```python
from build123d import *

# Parameters (mm, degrees)
F0_W      = 279.4
F0_H      = 44.45
F1_DEPTH  = 31.75
F2_W      = 165.1
F2_H      = 38.1
F3_DEPTH  = 28.575
F5_DEPTH  = 31.751
F6_W      = 6.35
F6_H      = 44.45
F7_DEPTH  = 31.75
F8_R      = 9.525
F9_R      = 5.588
F10_R     = 2.54
F11_DEPTH = 279.4
F12_W     = 25.4
F12_H     = 28.575
F12_H_2   = 12.7
F13_DEPTH = 31.751
F14_R     = 2.54
F15_DEPTH = 7.62
F16_R     = 7.9375
F17_R     = 5.08
F18_R     = 4.7625
F19_DEPTH = 17.272
F20_R     = 4.7625
F21_DEPTH = 17.272
F22_R     = 1.984375
F23_DEPTH = 41.91
F24_R     = 1.5875
F25_DEPTH = 3.175


with BuildPart() as f1:
    # F0 (on Top) → F1 (new body)
    with BuildSketch(Plane.XY):
        with Locations((139.7, 22.225)):
            Rectangle(F0_W, F0_H)
    extrude(amount=F1_DEPTH)

    # F2 (on face) → F3 (cut)
    with BuildSketch(Plane.XY.offset(31.75)):
        with Locations((139.7, 22.225)):
            Rectangle(F2_W, F2_H)
    extrude(amount=-F3_DEPTH, mode=Mode.SUBTRACT)

    # F4 (on face) → F5 (cut, through all)
    with BuildSketch(Plane(origin=(0, 0, 0), x_dir=(1, 0, 0), z_dir=(0, 0, -1))):
        with BuildLine():
            Line((127, -26.035), (209.867099, -26.025243))
            ThreePointArc((209.867099, -26.025243), (213.405749, -22.066069), (209.55, -18.415))
            Line((209.55, -18.415), (127, -18.415))
            ThreePointArc((127, -18.415), (123.19, -22.225), (127, -26.035))
        make_face()
    extrude(amount=-F5_DEPTH, mode=Mode.SUBTRACT)

    # F6 (on face) → F7 (join)
    with BuildSketch(Plane.XY.offset(31.75)):
        with Locations((3.175, 22.225)):
            Rectangle(F6_W, F6_H)
        with Locations((276.225, 22.225)):
            Rectangle(F6_W, F6_H)
    extrude(amount=F7_DEPTH)

    # F8
    f8_edges = [f1.edges().sort_by_distance(p)[0] for p in [
        (57.15, 3.175, 17.4625),
        (57.15, 41.275, 17.4625),
        (222.25, 3.175, 17.4625),
        (222.25, 41.275, 17.4625),
    ]]
    fillet(f8_edges, radius=F8_R)

    # F9
    f9_edges = [f1.edges().sort_by_distance(p)[0] for p in [
        (0, 44.45, 31.75),
        (0, 0, 31.75),
        (279.4, 44.45, 31.75),
        (279.4, 0, 31.75),
    ]]
    fillet(f9_edges, radius=F9_R)

    # F10 (on Right) → F11 (cut)
    with BuildSketch(Plane.YZ):
        with Locations((22.225, 54.61)):
            Circle(F10_R)
    extrude(amount=F11_DEPTH, mode=Mode.SUBTRACT)

    # F12 (on face) → F13 (cut, through all)
    with BuildSketch(Plane.XY.offset(31.75)):
        with Locations((28.575, 22.225)):
            Rectangle(F12_W, F12_H)
        with Locations((247.65, 22.225)):
            Rectangle(F12_W, F12_H_2)
    extrude(amount=-F13_DEPTH, mode=Mode.SUBTRACT)

    # F14 (on Right) → F15 (cut)
    with BuildSketch(Plane.YZ):
        with Locations((22.225, 34.925)):
            Circle(F14_R)
    extrude(amount=F15_DEPTH, mode=Mode.SUBTRACT)

    # F16
    f16_edges = [f1.edges().sort_by_distance(p)[0] for p in [
        (15.875, 36.5125, 15.875),
        (41.275, 36.5125, 15.875),
        (41.275, 7.9375, 15.875),
        (15.875, 7.9375, 15.875),
    ]]
    fillet(f16_edges, radius=F16_R)

    # F17
    f17_edges = [f1.edges().sort_by_distance(p)[0] for p in [
        (234.95, 28.575, 15.875),
        (260.35, 28.575, 15.875),
        (260.35, 15.875, 15.875),
        (234.95, 15.875, 15.875),
    ]]
    fillet(f17_edges, radius=F17_R)

    # F18 (on face) → F19 (join)
    with BuildSketch(Plane.XZ):
        with Locations((177.8, 9.525)):
            Circle(F18_R)
        with Locations((74.295, 19.05)):
            Circle(F18_R)
    extrude(amount=-F19_DEPTH)

    # F20 (on face) → F21 (join)
    with BuildSketch(Plane(origin=(0, 44.45, 0), x_dir=(-1, 0, 0), z_dir=(0, 1, 0))):
        with Locations((-177.8, 9.525)):
            Circle(F20_R)
        with Locations((-74.295, 19.05)):
            Circle(F20_R)
    extrude(amount=-F21_DEPTH)

    # F22 (on face) → F23 (cut)
    with BuildSketch(Plane.XZ):
        with Locations((74.307166, 19.073443)):
            Circle(F22_R)
        with Locations((177.807808, 9.510602)):
            Circle(F22_R)
    extrude(amount=-F23_DEPTH, mode=Mode.SUBTRACT)

    # F24 (on face) → F25 (cut)
    with BuildSketch(Plane(origin=(0, 44.45, 0), x_dir=(-1, 0, 0), z_dir=(0, 1, 0))):
        with Locations((-177.769601, 9.552136)):
            Circle(F24_R)
        with Locations((-74.274786, 19.058295)):
            Circle(F24_R)
    extrude(amount=-F25_DEPTH, mode=Mode.SUBTRACT)


solid = f1.part
```
The listing builds one solid part. Answer for the finished solid, in the listing's coordinates (mm). A direction names the side the tool comes from. Round coordinates to 2 decimals unless told otherwise and drop trailing zeros. Loops run counter-clockwise (first coordinate to the right, second up) from the corner with the lowest first, then second, coordinate; pieces in that order, holes last.
Q1. Given pin 1 Ø19 at (x, y) = (138, 31) entering from +Z (3 decimals); pin 2 Ø4.5 at (x, z) = (74.31, 19.07) entering from -Y, each flat-ended and moving along its own axis, determine where each tip first touches the part or whether it passes through.
Q2. For a pull along X with two mould halves and no side action, classify faces 6 (the face through (3.131, 20.209, 53.064)), 7 (the face through (15.875, 22, 16)), 8 (the face through (0, 22, 31)) as released by +X, released by -X, zero draft, split by the parting line, or undercut.
Q3. Which of the six approach directions +Z, -Z, +X, -X, +Y, -Y give full straight-line access (tool end or side, diameter ignored) to faces 1 (the face through (29, 7.938, 16)), 2 (the face through (138, 3, 31.75)), 3 (the face through (76.3, 17.272, 18.1)), 4 (the face through (182.2, 10.1, 7.7)), 5 (the face through (279.4, 22, 31))?
Q4. Section D-D, the plane x = 164.5 is taken. Determine the outline of the cut face in (y, z) (3 decimals).
Q5. Section B-B, the plane z = 42 is taken. Determine the outline of the cut face in (x, y).
Q6. Section A-A, the plane z = 54.61 is taken. Determine the outline of the cut face in (x, y) (3 decimals).
Q7. Section C-C, the plane x = 114.5 is taken. Determine the outline of the cut face in (y, z) (3 decimals).
Q8. Find the intervals of material crossed by line 1 (X direction, y = 24, z = 4) (3 decimals); line 2 (X direction, y = 30, z = 40.5); line 3 (Y direction, x = 135.5, z = 23.5) (3 decimals), in increasing order.
Completed:
1. pin 1: stops at z = 3.175
1. pin 2: stops at y = 0
2. face 6: zero draft
2. face 7: undercut
2. face 8: released by -X
3. face 1: +Z, -Z
3. face 2: +Z, +Y, -Y
3. face 3: +Z
3. face 4: none
3. face 5: +Z, -Z, +X, +Y, -Y
4. outline: (0, 0) - (18.415, 0) - (18.415, 3.175) - (3.175, 3.175) - (3.175, 31.75) - (0, 31.75) - close; (26.031, 0) - (44.45, 0) - (44.45, 31.75) - (41.275, 31.75) - (41.275, 3.175) - (26.031, 3.175) - close
5. outline: (0, 5.59) arc R5.59 ccw to (5.59, 0) - (6.35, 0) - (6.35, 44.45) - (5.59, 44.45) arc R5.59 ccw to (0, 38.86) - close; (273.05, 0) - (273.81, 0) arc R5.59 ccw to (279.4, 5.59) - (279.4, 38.86) arc R5.59 ccw to (273.81, 44.45) - (273.05, 44.45) - close
6. outline: (0, 5.588) arc R5.588 ccw to (5.588, 0) - (6.35, 0) - (6.35, 19.685) - (0, 19.685) - close; (0, 24.765) - (6.35, 24.765) - (6.35, 44.45) - (5.588, 44.45) arc R5.588 ccw to (0, 38.862) - close; (273.05, 0) - (273.812, 0) arc R5.588 ccw to (279.4, 5.588) - (279.4, 19.685) - (273.05, 19.685) - close; (273.05, 24.765) - (279.4, 24.765) - (279.4, 38.862) arc R5.588 ccw to (273.812, 44.45) - (273.05, 44.45) - close
7. outline: (0, 0) - (44.45, 0) - (44.45, 31.75) - (41.275, 31.75) - (41.275, 3.175) - (3.175, 3.175) - (3.175, 31.75) - (0, 31.75) - close
8. line 1: x = 0 to 15.875, 41.275 to 57.15, 222.25 to 234.975, 260.325 to 279.4
8. line 2: x = 0 to 6.35, 273.05 to 279.4
8. line 3: y = 0 to 3.175, 41.275 to 44.45
